Input: part model. Units: mm. Frame: model coordinates. A direction names the side the tool comes from. Give positions to 0.01 mm unless a question says otherwise; leave off trailing zeros. Order: outer loops, then holes, each group sorted by start corner. A loop starts at its lowest first (then second) coordinate and runs counter-clockwise, first axis right, second up. Notation, with made-up numbers: M 49.25,13.5 L 94.25,13.5 A24 ccw 94.25,34.5 Z; hole C -18,24 d8. An arc over 180 degrees is marked long. Use a Markdown table: item, result.
from build123d import *

# Parameters (mm, degrees)
SKETCH_W        = 50
SKETCH_H        = 20
SKETCH_R        = 2.1
PAD_DEPTH       = 22
SKETCH001_R     = 11.2
POCKET_DEPTH    = 8
SKETCH002_R     = 5.1
SKETCH002_R_2   = 1.75
POCKET001_DEPTH = 20
CHAMFER_SIZE    = 1
FILLET_R        = 2
CHAMFER001_SIZE = 1
FILLET001_R     = 1
CHAMFER002_SIZE = 0.4


with BuildPart() as part:
    # Sketch → Pad (new body)
    with BuildSketch(Plane.XY):
        with Locations((25, 10)):
            Rectangle(SKETCH_W, SKETCH_H)
        with Locations((10, 15)):
            Circle(SKETCH_R, mode=Mode.SUBTRACT)
        with Locations((10, 5)):
            Circle(SKETCH_R, mode=Mode.SUBTRACT)
        with Locations((40, 15)):
            Circle(SKETCH_R, mode=Mode.SUBTRACT)
        with Locations((40, 5)):
            Circle(SKETCH_R, mode=Mode.SUBTRACT)
    extrude(amount=PAD_DEPTH)

    # Sketch001 (on Face3 of Pad) → Pocket (cut)
    with BuildSketch(Plane.XZ):
        with Locations((25, 11)):
            Circle(SKETCH001_R)
    extrude(amount=-POCKET_DEPTH, mode=Mode.SUBTRACT)

    # Sketch002 (on Face1 of Pocket) → Pocket001 (cut)
    with BuildSketch(Plane(origin=(0, 20, 0), x_dir=(-1, 0, 0), z_dir=(0, 1, 0))):
        with Locations((-25, 11)):
            Circle(SKETCH002_R)
        with Locations((-25, 18.95)):
            Circle(SKETCH002_R_2)
        with Locations((-25, 3.05)):
            Circle(SKETCH002_R_2)
        with Locations((-32.95, 11)):
            Circle(SKETCH002_R_2)
        with Locations((-17.05, 11)):
            Circle(SKETCH002_R_2)
    extrude(amount=-POCKET001_DEPTH, mode=Mode.SUBTRACT)

    # Chamfer
    chamfer_edges = [part.edges().sort_by_distance(p)[0] for p in [
        (13.8, 0, 11),
        (33.632493, 0, 18.13583),
    ]]
    chamfer(chamfer_edges, length=CHAMFER_SIZE)

    # Fillet
    fillet_edges = [part.edges().sort_by_distance(p)[0] for p in [
        (22.892869, 4.5, 0),
        (27.107131, 4.5, 0),
        (22.892869, 4.5, 22),
        (27.107131, 4.5, 22),
    ]]
    fillet(fillet_edges, radius=FILLET_R)

    # Chamfer001
    chamfer001_edges = [part.edges().sort_by_distance(p)[0] for p in [
        (7.671957, 0, 22),
        (0, 0, 11),
        (7.671957, 0, 0),
        (42.328043, 0, 0),
        (50, 0, 11),
        (42.328043, 0, 22),
    ]]
    chamfer(chamfer001_edges, length=CHAMFER001_SIZE)

    # Fillet001
    fillet001_edges = [part.edges().sort_by_distance(p)[0] for p in [
        (0, 10.5, 0),
        (50, 10.5, 0),
        (50, 10.5, 22),
        (0, 10.5, 22),
    ]]
    fillet(fillet001_edges, radius=FILLET001_R)

    # Chamfer002
    chamfer002_edges = [part.edges().sort_by_distance(p)[0] for p in [
        (49.707107, 20, 21.707107),
        (25, 20, 22),
        (0.292893, 20, 21.707107),
        (0, 20, 11),
        (0.292893, 20, 0.292893),
        (25, 20, 0),
        (49.707107, 20, 0.292893),
        (50, 20, 11),
    ]]
    chamfer(chamfer002_edges, length=CHAMFER002_SIZE)


solid = part.part
1) Mould query, pull axis X, two halves, no side actions, for faces 4 (the face through (25, 10, 0)), 5 (the face through (29.05, 14.08, 7.9)), 6 (the face through (33.709, 0.507, 0.828)), 7 (the face through (49.699, 10.286, 21.715)). Classes: released by +X, released by -X, zero draft, split by the parting line, or undercut.
Response values:
| item | result |
|---|---|
| face 4 | zero draft |
| face 5 | undercut |
| face 6 | undercut |
| face 7 | released by +X |
2) Cut plane C-C on x = 40. Return loops of the section in (y, z).
Response values:
| item | result |
|---|---|
| outline | M 0,1 L 1,0 L 2.9,0 L 2.9,22 L 1,22 L 0,21 Z; M 7.1,0 L 12.9,0 L 12.9,22 L 7.1,22 Z; M 17.1,0 L 19.6,0 L 20,0.4 L 20,21.6 L 19.6,22 L 17.1,22 Z |
3) Reachability of faces 1 (the face through (7.9, 5.09, 10.85)), 2 (the face through (13.8, 4.5, 11.1)), 3 (the face through (16.27, 0.51, 21.19)) from +Z, -Z, +X, -X, +Y, -Y: full face, straight path, thin tool, end or side. Return the list, or none.
Response values:
| item | result |
|---|---|
| face 1 | +Z, -Z |
| face 2 | -Y |
| face 3 | +Z, -Y |
4) Cut plane B-B on y = 15. Return loops of the section in (x, z).
Response values:
| item | result |
|---|---|
| outline | M 0,1 A1 ccw 1,0 L 7.9,0 L 7.9,22 L 1,22 A1 ccw 0,21 Z; M 12.1,0 L 37.9,0 L 37.9,22 L 12.1,22 Z; M 42.1,0 L 49,0 A1 ccw 50,1 L 50,21 A1 ccw 49,22 L 42.1,22 Z; hole C 17.05,11 d3.5; hole C 25,11 d10.2; hole C 25,3.05 d3.5; hole C 25,18.95 d3.5; hole C 32.95,11 d3.5 |
5) First-contact query: pin 1 Ø4 at (x, z) = (25, 3.05) entering from -Y. Flat tip, straight axial feed; report the tip coordinate or a pass-through.
Response values:
| item | result |
|---|---|
| pin 1 | stops at y = 8 |
6) Cut plane D-D on y = 10.75. Return loops of the section in (x, z), and give its area (3 significant figures).
Response values:
| item | result |
|---|---|
| outline | M 0,1 A1 ccw 1,0 L 49,0 A1 ccw 50,1 L 50,21 A1 ccw 49,22 L 1,22 A1 ccw 0,21 Z; hole C 17.05,11 d3.5; hole C 25,11 d10.2; hole C 25,3.05 d3.5; hole C 25,18.95 d3.5; hole C 32.95,11 d3.5 |
| area | 979 mm² |
7) Cut plane A-A on z = 11. State how many separate pieces and enclosed holes the cut face has, and give its area (3 significant figures).
Response values:
| item | result |
|---|---|
| separate pieces | 4 |
| enclosed holes | 4 |
| area | 557 mm² |
8) Material intervals for line 1 (Y direction, x = 40, z = 14.5); line 2 (Z direction, x = 25, y = 14.5); line 3 (Z direction, x = 17, y = 16.5), sorted ascending. Write a range as from..to.
Response values:
| item | result |
|---|---|
| line 1 | y = 0..2.9, 7.1..12.9, 17.1..20 |
| line 2 | z = 0..1.3, 4.8..5.9, 16.1..17.2, 20.7..22 |
| line 3 | z = 0..9.25, 12.75..22 |
